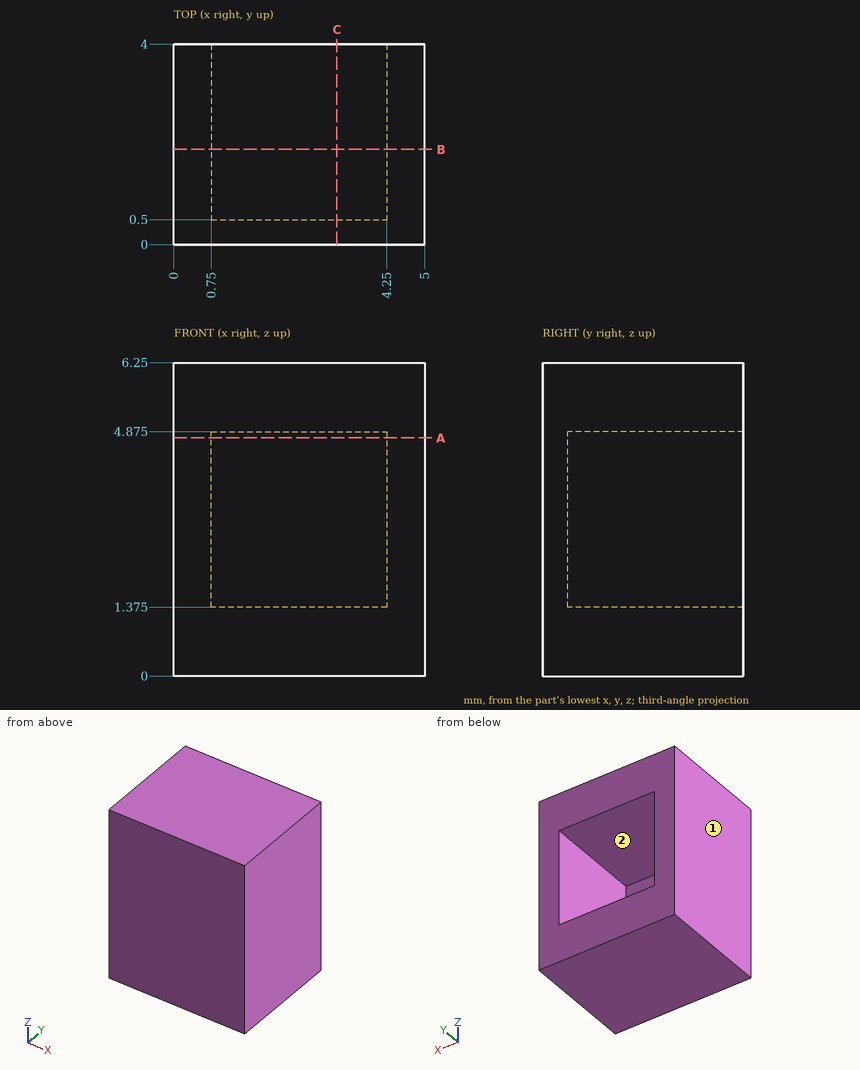
Design review of the part shown in the three views and the two pictorial views. Dimensions are in mm from the part's minimum x, y and z. A direction names the side the tool comes from. Coordinates: 2 decimals unless noted, no trailing zeros. Order: outer loops, then holes, each group sorted by start corner. A loop starts at its lowest first (then second) coordinate and runs counter-clockwise, first axis right, second up. Notation, with made-up numbers: (32, -16.5) -> (71, -16.5) arc R18 cw to (71, 9.5) -> close; hole circle Ø11 at (47.5, 7). An arc over 180 degrees is marked (long way). Use one line per item in the form item = value. Start each with the question number.
(1) Add section B-B on y = 1.9. State the section outline as (x, z) points (3 decimals), plus the area to 3 significant figures.
(2) For the marked faces 1 and 2, list the 3-axis set-ups (+Z, -Z, +X, -X, +Y, -Y) from which the entire face can be reached by the end or side of a thin tool; tool diameter is ignored.
(3) For probe 1 along Z at (x, y) = (3.35, 1.7) (3 decimals); probe 2 along X at (y, z) = (3.4, 4); probe 3 along Y at (x, z) = (2.5, 2.5), list the stretches that pass through material, from the lowest coordinate up.
(4) Add section A-A on z = 4.75. State the section outline as (x, y) points.
(5) Add section C-C on x = 3.25. State the section outline as (y, z) points (3 decimals).
Answer block:
q1.outline = (0, 0) -> (5, 0) -> (5, 6.25) -> (0, 6.25) -> close; hole (0.75, 1.375) -> (4.25, 1.375) -> (4.25, 4.875) -> (0.75, 4.875) -> close
q1.area = 19.0 mm²
q2.face_1 = +Z, -Z, -X, +Y, -Y
q2.face_2 = +Y
q3.probe_1 = 0 to 1.375, 4.875 to 6.25
q3.probe_2 = 0 to 0.75, 4.25 to 5
q3.probe_3 = 0 to 0.5
q4.outline = (0, 0) -> (5, 0) -> (5, 4) -> (4.25, 4) -> (4.25, 0.5) -> (0.75, 0.5) -> (0.75, 4) -> (0, 4) -> close
q5.outline = (0, 0) -> (4, 0) -> (4, 1.375) -> (0.5, 1.375) -> (0.5, 4.875) -> (4, 4.875) -> (4, 6.25) -> (0, 6.25) -> close
